Verification items for this drawing (mm, ordinates from the low corner). A direction names the side the tool comes from. Round coordinates to 2 decimals unless told otherwise and drop trailing zeros. Order: outer loops, then holes, each group sorted by start corner. A loop starts at its lowest first (then second) coordinate and runs counter-clockwise, first axis right, second up. Notation, with made-up numbers: (46, 84.25) -> (53, 84.25) arc R21 ccw to (53, 93.25) -> close; hole circle Ø11 at (60, 70). An arc over 180 degrees is marked (long way). Answer in a Markdown table with one row per item. Add a question column.
1. Sectioned sample at D-D, the plane z = 2.5. Record the boundary of the cut face in (x, y) (1 decimal), then the cut area to 3 significant figures.
2. Sectioned sample at B-B, the plane z = 10. Record the boundary of the cut face in (x, y) (1 decimal).
3. Material ranges on L1, parallel to Y at x = 4.5, z = 3.5; L2, parallel to Z at x = 20.5, y = 0.75; L3, parallel to Z at x = 20.5, y = 14.55, recorded low to high. Write a range as from..to.
4. Access from +Z, -Z, +X, -X, +Y, -Y to the whole of each face (thin tool, end or side, straight path). Record for the marked faces 1, 2, 3 and 4.
5. Sectioned sample at C-C, the plane x = 20.5. Record the boundary of the cut face in (y, z), then the cut area to 3 significant figures.
6. Depth check by flat-ended pin: P1, Ø10, axis at y = 6, z = 18, coming from the +X side; P2, Ø6, axis at x = 33.5, z = 6.5, coming from the -Y side; P3, Ø11.5, axis at x = 4.5, z = 14, coming from the -Y side. Enter the tip coordinate at first touch or a pass-through.
7. Draft check along Y on the marked faces 5, 6, 7 and 8. Enter one of: +Y half, -Y half, draft (parallel to the pull), parting line (faces both ways), or undercut.
8. Sectioned sample at A-A, the plane x = 5. Record the boundary of the cut face in (y, z), then the cut area to 3 significant figures.
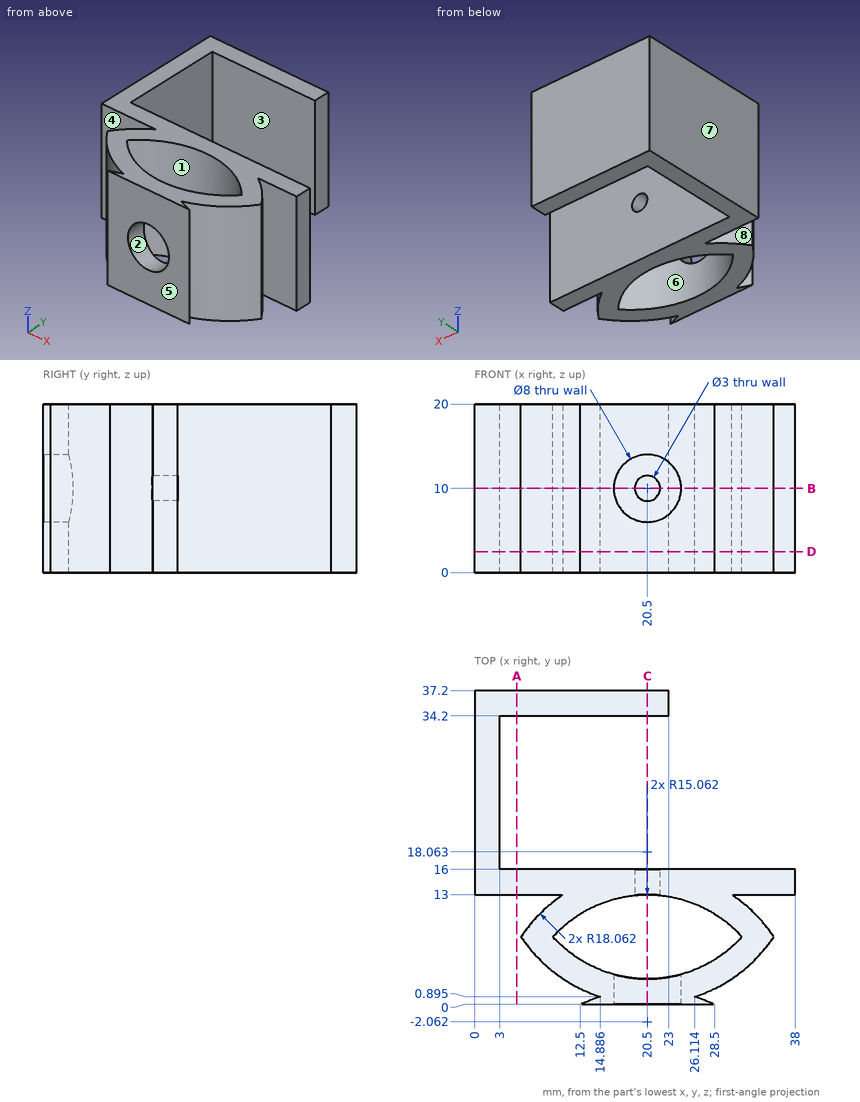
Answer key:
| question | item | result |
|---|---|---|
| 1 | outline | (0, 13) -> (10.5, 13) arc R18.1 ccw to (5.5, 8) arc R18.1 ccw to (14.9, 0.9) -> (12.5, 0) -> (28.5, 0) -> (26.1, 0.9) arc R18.1 ccw to (35.5, 8) arc R18.1 ccw to (30.5, 13) -> (38, 13) -> (38, 16) -> (3, 16) -> (3, 34.2) -> (23, 34.2) -> (23, 37.2) -> (0, 37.2) -> close; hole (9.3, 8) arc R15.1 ccw to (31.7, 8) arc R15.1 ccw to start |
| 1 | area | 385 mm² |
| 2 | outline | (0, 13) -> (10.5, 13) arc R18.1 ccw to (5.5, 8) arc R18.1 ccw to (14.9, 0.9) -> (12.5, 0) -> (16.5, 0) -> (16.5, 3.5) arc R15.1 cw to (9.3, 8) arc R15.1 cw to (19, 12.9) -> (19, 16) -> (3, 16) -> (3, 34.2) -> (23, 34.2) -> (23, 37.2) -> (0, 37.2) -> close; (22, 12.9) arc R15.1 cw to (31.7, 8) arc R15.1 cw to (24.5, 3.5) -> (24.5, 0) -> (28.5, 0) -> (26.1, 0.9) arc R18.1 ccw to (35.5, 8) arc R18.1 ccw to (30.5, 13) -> (38, 13) -> (38, 16) -> (22, 16) -> close |
| 3 | L1 | y = 13..16, 34.2..37.2 |
| 3 | L2 | z = 0..6, 14..20 |
| 3 | L3 | z = 0..8.5, 11.5..20 |
| 4 | face 1 | +Z, -Z |
| 4 | face 2 | -Y |
| 4 | face 3 | +Z, -Z, +X |
| 4 | face 4 | +Z, -Z, -X |
| 5 | outline | (0, 0) -> (3, 0) -> (3, 6) -> (0, 6) -> close; (0, 14) -> (3, 14) -> (3, 20) -> (0, 20) -> close; (13, 0) -> (16, 0) -> (16, 8.5) -> (13, 8.5) -> close; (13, 11.5) -> (16, 11.5) -> (16, 20) -> (13, 20) -> close; (34.2, 0) -> (37.2, 0) -> (37.2, 20) -> (34.2, 20) -> close |
| 5 | area | 147 mm² |
| 6 | P1 | stops at x = 35.5 |
| 6 | P2 | stops at y = 3.02 |
| 6 | P3 | stops at y = 3.19 |
| 7 | face 5 | -Y half |
| 7 | face 6 | undercut |
| 7 | face 7 | draft |
| 7 | face 8 | undercut |
| 8 | outline | (13, 0) -> (16, 0) -> (16, 20) -> (13, 20) -> close; (34.2, 0) -> (37.2, 0) -> (37.2, 20) -> (34.2, 20) -> close |
| 8 | area | 120 mm² |
